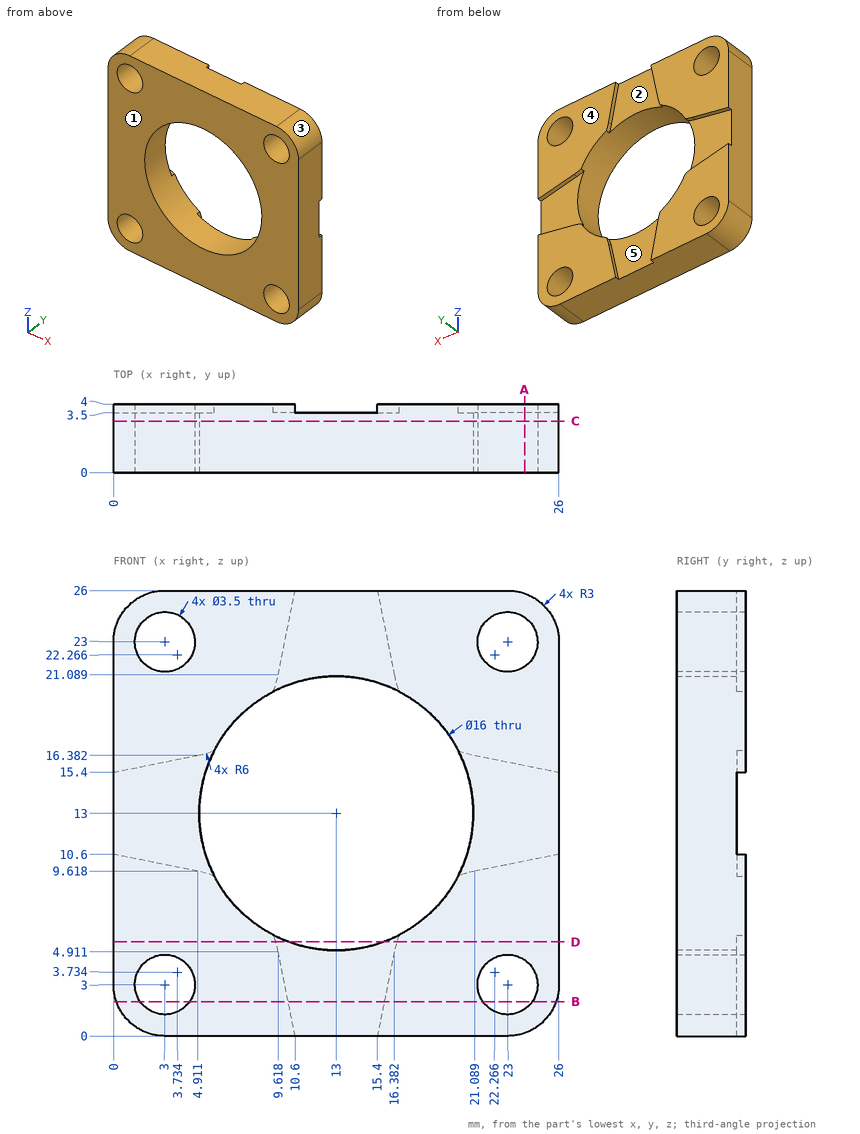
Study the drawing (mm; zero at the part's minimum x, y, z) and answer. A direction names the side the tool comes from. Round coordinates to 2 decimals unless told otherwise and drop trailing zeros. Write each loop counter-clockwise with the first axis right and the second up, starting at its lowest first coordinate (ties: lowest second). Pieces come first, ordered by that corner, then holes. Notation, with made-up numbers: (-22, 47.25) -> (35, 47.25) arc R13 ccw to (35, 55.25) -> close; hole circle Ø5 at (17.25, 20.5). An arc over 180 degrees is marked (long way). Write item = value, one per line.
1) For a pull along X with two mould halves and no side action, classify the marked faces 1, 2 and 3 as released by +X, released by -X, zero draft, split by the parting line, or undercut.
Check values:
face_1 = zero draft
face_2 = undercut
face_3 = released by +X
2) Section D-D on z = 5.5 is taken. Write down the section's boundary in (x, y).
Check values:
outline = (0, 0) -> (10.22, 0) -> (10.22, 3.5) -> (9.47, 3.5) -> (9.47, 4) -> (0, 4) -> close; (15.78, 0) -> (26, 0) -> (26, 4) -> (16.53, 4) -> (16.53, 3.5) -> (15.78, 3.5) -> close
3) Section B-B on z = 2 is taken. Write down the section's boundary in (x, y).
Check values:
outline = (0.17, 0) -> (1.56, 0) -> (1.56, 4) -> (0.17, 4) -> close; (4.44, 0) -> (21.56, 0) -> (21.56, 4) -> (15.8, 4) -> (15.8, 3.5) -> (10.2, 3.5) -> (10.2, 4) -> (4.44, 4) -> close; (24.44, 0) -> (25.83, 0) -> (25.83, 4) -> (24.44, 4) -> close
4) Which of the six approach directions +Z, -Z, +X, -X, +Y, -Y give full straight-line access (tool end or side, diameter ignored) to the marked faces 4 and 5?
Check values:
face_4 = +Z, -Z, +X, -X, +Y
face_5 = +Y
5) Given pin 1 (3 mm diameter, centred on x = 3, z = 3, fed in from -Y); pin 2 (3 mm diameter, centred on x = 3.5, z = 14, fed in from +Y), each flat-ended and moving along its own axis, determine where each tip first touches the part or whether it passes through.
Check values:
pin_1 = through
pin_2 = 3.5
6) Section C-C on y = 3 is taken. Write down the section's boundary in (x, z).
Check values:
outline = (0, 3) arc R3 ccw to (3, 0) -> (23, 0) arc R3 ccw to (26, 3) -> (26, 23) arc R3 ccw to (23, 26) -> (3, 26) arc R3 ccw to (0, 23) -> close; hole circle Ø3.5 at (3, 3); hole circle Ø3.5 at (3, 23); hole circle Ø16 at (13, 13); hole circle Ø3.5 at (23, 3); hole circle Ø3.5 at (23, 23)
7) Straight lines are drawn through the part: line 1 along X through (y, z) = (2.55, 3); line 2 along Z through (x, y) = (13, 2.4). For each, find the intervals that lie inside material, in ascending order. Write a range as [from, to].
Check values:
line_1 = [0, 1.25], [4.75, 21.25], [24.75, 26]
line_2 = [0, 5], [21, 26]
8) Section A-A on x = 24 is taken. Write down the section's boundary in (y, z).
Check values:
outline = (0, 0.17) -> (4, 0.17) -> (4, 1.56) -> (0, 1.56) -> close; (0, 4.44) -> (4, 4.44) -> (4, 10.2) -> (3.5, 10.2) -> (3.5, 15.8) -> (4, 15.8) -> (4, 21.56) -> (0, 21.56) -> close; (0, 24.44) -> (4, 24.44) -> (4, 25.83) -> (0, 25.83) -> close
